from build123d import *

# Parameters (mm, degrees)
SKETCH_1_R      = 1.45
EXTRUDE_1_DEPTH = 5
CHAMFER_1_SIZE  = 0.5


with BuildPart() as part:
    # 스케치1 → 보스-돌출1 (new body)
    with BuildSketch(Plane.XY):
        Circle(SKETCH_1_R)
    extrude(amount=EXTRUDE_1_DEPTH)

    # 스케치3 → 회전1 (revolve)
    with BuildSketch(Plane(origin=(0, 0, 0), x_dir=(0, 0, -1), z_dir=(1, 0, 0)), mode=Mode.PRIVATE) as revolve_1_sk:
        Polygon((0, 0), (3, 0), (3, -2), (1.5, -3.5), (-2.05, -3.5), (0, -1.45), align=None)
    revolve(revolve_1_sk.sketch.rotate(Axis((0, 0, 0), (0, 0, -1)), 270), axis=Axis((0, 0, 0), (0, 0, -1)))

    # 모따기1
    chamfer_1_edges = [part.edges().sort_by_distance(p)[0] for p in [
        (-1.45, 0, 5),
    ]]
    chamfer(chamfer_1_edges, length=CHAMFER_1_SIZE)


solid = part.part
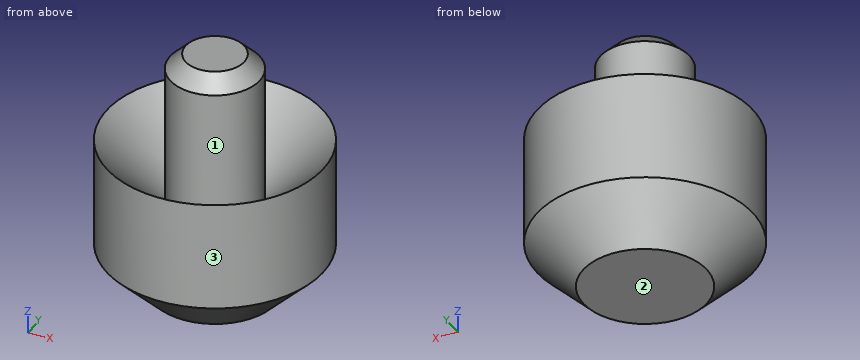
The listing builds one solid part. Answer for the finished solid, in the listing's coordinates (mm). Face numbers are marked on the shaded views. Round coordinates to 2 decimals unless told otherwise and drop trailing zeros. Order: outer loops, then holes, each group sorted by start corner. A loop starts at its lowest first (then second) coordinate and runs counter-clockwise, first axis right, second up. Notation, with made-up numbers: M 84.25,-13.5 L 125.25,-13.5 A18 cw 125.25,-2.5 Z; hole C 66.25,0.5 d3. An arc over 180 degrees is marked long. Answer in a Markdown table with one row per item. Add a question column.
1) The part is cut by section B-B on x = 0. Determine the outline of the cut face in (y, z), plus the area to 3 significant figures.
2) The part is cut by section A-A on z = 1.5. Determine the outline of the cut face in (x, y).
3) Flat-ended cylindrical pins translate along their axes: pin 1 Ø2 at (x, z) = (1.5, 3.5) entering from -Y; pin 2 Ø2 at (x, y) = (1, 2.5) entering from +Z; pin 3 Ø1 at (y, z) = (0.5, 3.5) entering from -X. Find the tip coordinate at first contact, or state that the pin passes through.
4) Determine the mould class of the marked faces 1, 2 and 3 for opening direction Y: pulls with the +Y half, pulls with the -Y half, needs draft (parallel to the pull), parting line crosses it, or undercut.
5) Consider line 1 along X through (y, z) = (-0.5, 1.75); line 2 along Y through (x, z) = (0.75, 0.25); line 3 along Y through (x, z) = (2.5, 1.5). Determine where each line is inside the solid, lowest interval first. Write a range as from..to.
6) The part is cut by section D-D on z = 2.5. Determine the outline of the cut face in (x, y), plus the area to 3 significant figures.
Findings below:
| question | item | result |
|---|---|---|
| 1 | outline | M -3.5,-1.5 L -2,-3 L 2,-3 L 3.5,-1.5 L 3.5,2.05 L 1.45,0 L 1.45,4.5 L 0.95,5 L -0.95,5 L -1.45,4.5 L -1.45,0 L -3.5,2.05 Z |
| 1 | area | 37.2 mm² |
| 2 | outline | C 0,0 d7; C 0,0 d2.9; hole C 0,0 d5.9 |
| 3 | pin 1 | stops at y = -1.36 |
| 3 | pin 2 | stops at z = 2.05 |
| 3 | pin 3 | stops at x = -1.45 |
| 4 | face 1 | undercut |
| 4 | face 2 | needs draft |
| 4 | face 3 | parting line crosses it |
| 5 | line 1 | x = -3.46..-3.16, -1.36..1.36, 3.16..3.46 |
| 5 | line 2 | y = -3.42..-1.53, -1.24..1.24, 1.53..3.42 |
| 5 | line 3 | y = -2.45..-1.57, 1.57..2.45 |
| 6 | outline | C 0,0 d2.9 |
| 6 | area | 6.61 mm² |
